Could you check a few things on this model? Use its own coordinates, in mm. A direction names the side the tool comes from. Round coordinates to 2 decimals unless told otherwise and drop trailing zeros. Order: outer loops, then holes, each group sorted by start corner. A loop starts at its lowest first (then second) coordinate and runs counter-clockwise, first axis right, second up. Notation, with made-up numbers: (52.5, -38) -> (65.5, -38) arc R32 ccw to (65.5, 1) -> close; hole circle Ø9 at (22.25, -4.5). An arc over 180 degrees is marked (long way). Put each result on its own line as item: value. Start each with the question number.
from build123d import *

# Parameters (mm, degrees)
BOSS_EXTRUDE1_DEPTH = 2.9718


with BuildPart() as part:
    # Sketch2 → Boss-Extrude1 (new body)
    with BuildSketch(Plane(origin=(0, 0, 0), x_dir=(0, 0, -1), z_dir=(1, 0, 0))):
        with BuildLine():
            Line((-73.009928621, 43.676956522), (53.990071379, 43.676956522))
            Line((53.990071379, 43.676956522), (53.990071379, 39.104956522))
            Line((53.990071379, 39.104956522), (50.942071379, 39.104956522))
            Line((50.942071379, 39.104956522), (50.942071379, 36.818956522))
            Line((50.942071379, 36.818956522), (47.989076338, 36.818956522))
            Line((47.989076338, 36.818956522), (47.989076338, 38.469956522))
            Line((47.989076338, 38.469956522), (45.100071379, 38.469956522))
            Line((45.100071379, 38.469956522), (45.100071379, 36.818956522))
            Line((45.100071379, 36.818956522), (41.036071379, 36.818956522))
            Line((41.036071379, 36.818956522), (41.036071379, 33.770956522))
            Line((41.036071379, 33.770956522), (45.100071379, 33.770956522))
            Line((45.100071379, 33.770956522), (45.100071379, 32.119956522))
            Line((45.100071379, 32.119956522), (47.989076338, 32.119956522))
            Line((47.989076338, 32.119956522), (47.989076338, 33.770956522))
            Line((47.989076338, 33.770956522), (50.942071379, 33.770956522))
            Line((50.942071379, 33.770956522), (50.942071379, 31.484956522))
            Line((50.942071379, 31.484956522), (53.990071379, 31.484956522))
            Line((53.990071379, 31.484956522), (53.990071379, -33.031043478))
            Line((53.990071379, -33.031043478), (50.942071379, -33.031043478))
            Line((50.942071379, -33.031043478), (50.942071379, -35.317043478))
            Line((50.942071379, -35.317043478), (47.989076338, -35.317043478))
            Line((47.989076338, -35.317043478), (47.989076338, -33.666043478))
            Line((47.989076338, -33.666043478), (45.100071379, -33.666043478))
            Line((45.100071379, -33.666043478), (45.100071379, -35.317043478))
            Line((45.100071379, -35.317043478), (41.036071379, -35.317043478))
            Line((41.036071379, -35.317043478), (41.036071379, -38.365043478))
            Line((41.036071379, -38.365043478), (45.100071379, -38.365043478))
            Line((45.100071379, -38.365043478), (45.100071379, -40.016043478))
            Line((45.100071379, -40.016043478), (47.989076338, -40.016043478))
            Line((47.989076338, -40.016043478), (47.989076338, -38.365043478))
            Line((47.989076338, -38.365043478), (50.942071379, -38.365043478))
            Line((50.942071379, -38.365043478), (50.942071379, -40.651043478))
            Line((50.942071379, -40.651043478), (53.990071379, -40.651043478))
            Line((53.990071379, -40.651043478), (53.990071379, -45.223043478))
            Line((53.990071379, -45.223043478), (-73.009928621, -45.223043478))
            Line((-73.009928621, -45.223043478), (-73.009928621, -40.651043478))
            Line((-73.009928621, -40.651043478), (-75.981728621, -40.651043478))
            Line((-75.981728621, -40.651043478), (-75.981728621, -37.179683686))
            ThreePointArc((-75.981728621, -37.179683686), (-72.971828621, -36.841043478), (-75.981728621, -36.502403271))
            Line((-75.981728621, -36.502403271), (-75.981728621, -33.031043478))
            Line((-75.981728621, -33.031043478), (-73.009928621, -33.031043478))
            Line((-73.009928621, -33.031043478), (-73.009928621, 31.484956522))
            Line((-73.009928621, 31.484956522), (-75.981728621, 31.484956522))
            Line((-75.981728621, 31.484956522), (-75.981728621, 34.956316314))
            ThreePointArc((-75.981728621, 34.956316314), (-72.971828621, 35.294956522), (-75.981728621, 35.633596729))
            Line((-75.981728621, 35.633596729), (-75.981728621, 39.104956522))
            Line((-75.981728621, 39.104956522), (-73.009928621, 39.104956522))
            Line((-73.009928621, 39.104956522), (-73.009928621, 43.676956522))
        make_face()
    extrude(amount=BOSS_EXTRUDE1_DEPTH)


solid = part.part
1. If we section it at B-B, the plane y = -15.5: Please give me the cut outline in (x, z), then the cut area to 3 significant figures.
2. For pin 1 Ø0.8 at (x, y) = (2, -39.5) entering from -Z; pin 2 Ø0.9 at (x, y) = (2, 35) entering from -Z; pin 3 Ø4 at (y, z) = (-25.5, 57.5) entering from -X; pin 4 Ø1.5 at (x, y) = (1, 29.5) entering from +Z, each with a flat end and sliding along its axis, tell me the tip position at first contact or that it passes through.
3. I need wall thicknesses on L1, parallel to Z at x = 1.45, y = 33.5; L2, parallel to Y at x = 2.15, z = -43.5; L3, parallel to Z at x = 1.7, y = 12.5. Which ranges of each line are inside material? Lowest first, please.
4. Which directions (+Z, -Z, +X, -X, +Y, -Y) give clear straight access to the entire face, cutting with the end or side of a thin tool? Please do faces 3 (the face through (1, 38.47, -47)), 4 (the face through (1, 41, 73.01)), 5 (the face through (1, 35, -41.036)).
5. Thinking about a two-plate mould opening in Y: for faces 1 (the face through (1, 0, -53.99)), 2 (the face through (1, -33.666, -47)), which applies, +Y half, -Y half, draft (parallel to the pull), parting line (faces both ways), or undercut?
6. If we section it at A-A, the plane z = -42.5: Please give me the cut outline in (x, y), then the cut area to 3 significant figures.
Results below:
1. outline: (0, -53.99) -> (2.97, -53.99) -> (2.97, 73.01) -> (0, 73.01) -> close
1. area: 377 mm2
2. pin 1: z = -50.94
2. pin 2: z = -41.04
2. pin 3: x = 0
2. pin 4: z = 73.01
3. L1: -50.94 to -47.99, -45.1 to 75.98
3. L2: -45.22 to -38.37, -35.32 to 33.77, 36.82 to 43.68
3. L3: -53.99 to 73.01
4. face 3: +X, -X
4. face 4: +Z, +X, -X, +Y
4. face 5: -Z, +X, -X
5. face 1: draft
5. face 2: undercut
6. outline: (0, -45.22) -> (2.97, -45.22) -> (2.97, -38.37) -> (0, -38.37) -> close; (0, -35.32) -> (2.97, -35.32) -> (2.97, 33.77) -> (0, 33.77) -> close; (0, 36.82) -> (2.97, 36.82) -> (2.97, 43.68) -> (0, 43.68) -> close
6. area: 246 mm2
